Geometry: final body of the model. Coordinates: model frame, mm. A direction names the side the tool comes from. Coordinates: 2 decimals unless noted, no trailing zeros. Loops run counter-clockwise (first coordinate to the right, second up) from the corner with the lowest first, then second, coordinate; pieces in that order, holes last. Notation, with made-up numbers: (38, 46.5) - (62, 46.5) arc R31 ccw to (62, 81.5) - close; hole circle Ø3 at (80.5, -26.5). An arc over 180 degrees is marked (long way). Answer in a Markdown table with one row per item.
from build123d import *

# Parameters (mm, degrees)
SKETCH1_W           = 25
SKETCH1_H           = 24
SKETCH1_R           = 1
BOSS_EXTRUDE1_DEPTH = 1.2
BOSS_EXTRUDE2_START = 1.2
BOSS_EXTRUDE2_DEPTH = 1.5
BOSS_EXTRUDE3_START = 1.2
SKETCH1_4_W         = 8.5
SKETCH1_4_H         = 8.5
BOSS_EXTRUDE3_DEPTH = 2
BOSS_EXTRUDE4_START = 1.2
SKETCH1_5_W         = 1.516820611
SKETCH1_5_H         = 0.819903033
SKETCH1_5_W_2       = 1.988264855
BOSS_EXTRUDE4_DEPTH = 1
SKETCH1_6_W         = 23
SKETCH1_6_H         = 4
SKETCH1_6_H_2       = 5
BOSS_EXTRUDE5_DEPTH = 2
BOSS_EXTRUDE6_START = 3.2
SKETCH1_7_R         = 4.25
BOSS_EXTRUDE6_DEPTH = 2
FILLET1_R           = 0.5


with BuildPart() as part:
    # Sketch1 → Boss-Extrude1 (new body)
    with BuildSketch(Plane(origin=(0, 0, 0), x_dir=(1, 0, 0), z_dir=(0, 1, 0))):
        with Locations((12.5, 12)):
            Rectangle(SKETCH1_W, SKETCH1_H)
        with Locations((2, 2)):
            Circle(SKETCH1_R, mode=Mode.SUBTRACT)
        with Locations((23, 2)):
            Circle(SKETCH1_R, mode=Mode.SUBTRACT)
        with Locations((2, 14.5)):
            Circle(SKETCH1_R, mode=Mode.SUBTRACT)
        with Locations((23, 14.5)):
            Circle(SKETCH1_R, mode=Mode.SUBTRACT)
    extrude(amount=BOSS_EXTRUDE1_DEPTH)

    # Sketch1<3> → Boss-Extrude2 (add)
    with BuildSketch(Plane(origin=(0, 0, 0), x_dir=(1, 0, 0), z_dir=(0, 1, 0)).offset(BOSS_EXTRUDE2_START)):
        Polygon((16.7, 10.25), (12.5, 10.25), (8.3, 10.25), (8.3, 2), (16.7, 2), align=None)
    extrude(amount=BOSS_EXTRUDE2_DEPTH)

    # Sketch1<4> → Boss-Extrude3 (add)
    with BuildSketch(Plane(origin=(0, 0, 0), x_dir=(1, 0, 0), z_dir=(0, 1, 0)).offset(BOSS_EXTRUDE3_START)):
        with Locations((12.5, 14.5)):
            Rectangle(SKETCH1_4_W, SKETCH1_4_H)
    extrude(amount=BOSS_EXTRUDE3_DEPTH)

    # Sketch1<5> → Boss-Extrude4 (add)
    with BuildSketch(Plane(origin=(0, 0, 0), x_dir=(1, 0, 0), z_dir=(0, 1, 0)).offset(BOSS_EXTRUDE4_START)):
        with Locations((4.706273263, 4.74063197)):
            Rectangle(SKETCH1_5_W, SKETCH1_5_H)
        with Locations((6.007869327, 3.469782269)):
            Rectangle(SKETCH1_5_W_2, SKETCH1_5_H)
    extrude(amount=BOSS_EXTRUDE4_DEPTH)

    # Sketch1<6> → Boss-Extrude5 (add)
    with BuildSketch(Plane(origin=(0, 0, 0), x_dir=(1, 0, 0), z_dir=(0, 1, 0))):
        with Locations((12.5, 22)):
            Rectangle(SKETCH1_6_W, SKETCH1_6_H)
        with Locations((12.5, 26.5)):
            Rectangle(SKETCH1_6_W, SKETCH1_6_H_2)
    extrude(amount=-BOSS_EXTRUDE5_DEPTH)

    # Sketch1<7> → Boss-Extrude6 (add)
    with BuildSketch(Plane(origin=(0, 0, 0), x_dir=(1, 0, 0), z_dir=(0, 1, 0)).offset(BOSS_EXTRUDE6_START)):
        with Locations((12.5, 14.5)):
            Circle(SKETCH1_7_R)
    extrude(amount=BOSS_EXTRUDE6_DEPTH)

    # Fillet1
    fillet1_edges = [part.edges().sort_by_distance(p)[0] for p in [
        (8.25, 5.2, -14.5),
    ]]
    fillet(fillet1_edges, radius=FILLET1_R)


solid = part.part
(1) Cut plane B-B on x = 17.5. Output: boundary loops of the cut face in (y, z), then the cut area to 3 significant figures.
Verdict:
| item | result |
|---|---|
| outline | (-2, -29) - (0, -29) - (0, -24) - (1.2, -24) - (1.2, 0) - (0, 0) - (0, -20) - (-2, -20) - close |
| area | 46.8 mm² |
(2) Cut plane C-C on z = -6.5. Output: boundary loops of the cut face in (x, y), then the cut area to 3 significant figures.
Verdict:
| item | result |
|---|---|
| outline | (0, 0) - (25, 0) - (25, 1.2) - (16.7, 1.2) - (16.7, 2.7) - (8.3, 2.7) - (8.3, 1.2) - (0, 1.2) - close |
| area | 42.6 mm² |
(3) Pull-direction query (X, two-part tool) for faces 4 (the face through (12, -1, -29)), 5 (the face through (7.002, 1.7, -3.5)), 6 (the face through (16.7, 2, -6)); classes: pulls with the +X half, pulls with the -X half, needs draft (parallel to the pull), parting line crosses it, or undercut.
Verdict:
| item | result |
|---|---|
| face 4 | needs draft |
| face 5 | undercut |
| face 6 | pulls with the +X half |
(4) Cut plane A-A on x = 2. Output: boundary loops of the cut face in (y, z).
Verdict:
| item | result |
|---|---|
| outline | (-2, -29) - (0, -29) - (0, -24) - (1.2, -24) - (1.2, -15.5) - (0, -15.5) - (0, -20) - (-2, -20) - close; (0, -13.5) - (1.2, -13.5) - (1.2, -3) - (0, -3) - close; (0, -1) - (1.2, -1) - (1.2, 0) - (0, 0) - close |
(5) Ray query, probe 1 along X at (y, z) = (0.85, -14.5); probe 2 along Z at (x, y) = (23, 0.4); probe 3 along Y at (x, z) = (11.25, -28). Return the intervals inside material, ascending.
Verdict:
| item | result |
|---|---|
| probe 1 | x = 0 to 1, 3 to 22, 24 to 25 |
| probe 2 | z = -24 to -15.5, -13.5 to -3, -1 to 0 |
| probe 3 | y = -2 to 0 |
(6) Cut plane D-D on y = -1.25. Output: boundary loops of the cut face in (x, z), then the cut area to 3 significant figures.
Verdict:
| item | result |
|---|---|
| outline | (1, -29) - (24, -29) - (24, -20) - (1, -20) - close |
| area | 207 mm² |
(7) Access query for faces 1 (the face through (9, 3.2, -18)), 2 (the face through (12, 2, -2)), 3 (the face through (5, 2.2, -5)). Directions: +Z, -Z, +X, -X, +Y, -Y. A direction counts if a zero-diameter tool reaches every point of the face in a straight line with its end or side. Return the directions, or none.
Verdict:
| item | result |
|---|---|
| face 1 | -Z, -X, +Y |
| face 2 | +Z, +X, -X, +Y |
| face 3 | +Z, -Z, -X, +Y |
(8) First-contact query: pin 1 Ø0.6 at (x, y) = (11.5, 2) entering from -Z; pin 2 Ø1.6 at (y, z) = (-1, -25) entering from -X; pin 3 Ø1.5 at (y, z) = (1.5, -25) entering from -X; pin 4 Ø0.6 at (x, y) = (17.5, -1.5) entering from +Z. Flat tips, straight axial feed; report the tip coordinate or a pass-through.
Verdict:
| item | result |
|---|---|
| pin 1 | stops at z = -18.75 |
| pin 2 | stops at x = 1 |
| pin 3 | passes through |
| pin 4 | stops at z = -20 |
